Read the model definition and answer for the solid it produces. Units are mm, in the model's axes. Face numbers are marked on the shaded views. A direction names the side the tool comes from. Coordinates: 2 decimals unless noted, no trailing zeros. Order: outer loops, then holes, each group sorted by start corner. A loop starts at its lowest first (then second) coordinate and runs counter-clockwise, first axis right, second up.
from build123d import *

# Parameters (mm, degrees)
F1_DEPTH = 29.9212
F2_DEPTH = 21.3614
F0_W     = 21.8694
F0_H     = 50.8
F3_DEPTH = 13.5636


with BuildPart() as f1:
    # F0 (on Top) → F1 (new body)
    with BuildSketch(Plane.XY):
        Polygon((-26.2128, -38.1), (-26.2128, 38.1), (-26.2128, 76.2), (-126.8476, 76.2), (-126.8476, -76.2), (-26.2128, -76.2), align=None)
    extrude(amount=F1_DEPTH)

    # F0 (on Top) → F2 (join)
    with BuildSketch(Plane.XY):
        Polygon((26.2128, 25.4), (26.2128, 38.1), (-26.2128, 38.1), (-26.2128, -38.1), (26.2128, -38.1), (26.2128, -25.4), align=None)
    extrude(amount=F2_DEPTH)

    # F0 (on Top) → F3 (join)
    with BuildSketch(Plane.XY):
        with Locations((37.1475, 0)):
            Rectangle(F0_W, F0_H)
    extrude(amount=F3_DEPTH)


solid = f1.part
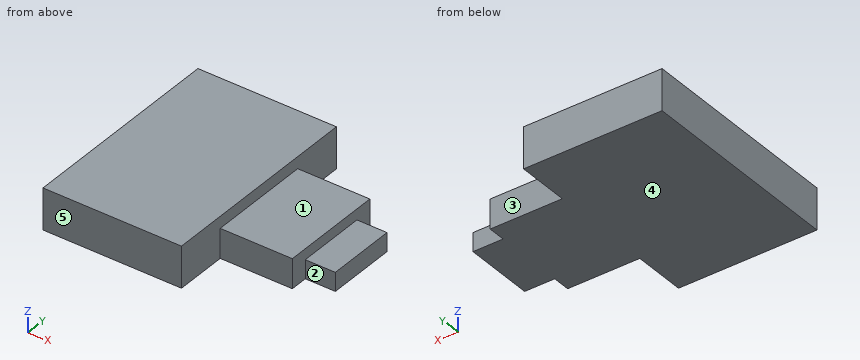
Q1. Which of the six approach directions +Z, -Z, +X, -X, +Y, -Y give full straight-line access (tool end or side, diameter ignored) to the marked faces 1, 2, 3, 4 and 5?
Q2. The part is cut by section A-A, the plane z = 6.25. Determine the outline of the cut face in (x, y).
Q3. The part is cut by section C-C, the plane x = 0. Determine the outline of the cut face in (y, z).
Q4. The part is cut by section B-B, the plane y = 14. Determine the outline of the cut face in (x, z), then the cut area to 3 significant figures.
Q5. Each of these flat-tipped pins is pushed along its axis until it touches: P1, Ø6.5, axis at x = 5, z = 12, coming from the -Y side; P2, Ø11, axis at x = 33, z = 5, coming from the -Y side; P3, Ø5, axis at x = -92, y = 18.5, coming from the -Z side; P4, Ø15, axis at x = 42.5, z = 8.5, coming from the +Y side. Where does it stop, or does it pass through?
Q6. Straight lines are drawn through the part: L1, parallel to Y at x = -14.5, z = 8.5; L2, parallel to X at y = 15, z = 16.75; L3, parallel to X at y = -70, z = 7. For each, find the intervals that lie inside material, in ascending order.
Q7. The part is cut by section D-D, the plane z = 26.5. Determine the outline of the cut face in (x, y).
Computed values:
1. face 1: +Z, +X, +Y, -Y
1. face 2: +Z, -Z, +X, -Y
1. face 3: +Z, -Z, +X, +Y
1. face 4: -Z, +X, -X, +Y, -Y
1. face 5: +Z, -Z, +X, -X, -Y
2. outline: (-126.85, -76.2) - (-26.21, -76.2) - (-26.21, -38.1) - (26.21, -38.1) - (26.21, -25.4) - (48.08, -25.4) - (48.08, 25.4) - (26.21, 25.4) - (26.21, 38.1) - (-26.21, 38.1) - (-26.21, 76.2) - (-126.85, 76.2) - close
3. outline: (-38.1, 0) - (38.1, 0) - (38.1, 21.36) - (-38.1, 21.36) - close
4. outline: (-126.85, 0) - (48.08, 0) - (48.08, 13.56) - (26.21, 13.56) - (26.21, 21.36) - (-26.21, 21.36) - (-26.21, 29.92) - (-126.85, 29.92) - close
4. area: 4,430 mm2
5. P1: stops at y = -38.1
5. P2: stops at y = -25.4
5. P3: stops at z = 0
5. P4: stops at y = 25.4
6. L1: y = -38.1 to 38.1
6. L2: x = -126.85 to 26.21
6. L3: x = -126.85 to -26.21
7. outline: (-126.85, -76.2) - (-26.21, -76.2) - (-26.21, 76.2) - (-126.85, 76.2) - close
